Could you check a few things on this model? Use its own coordinates, in mm. Round coordinates to 2 decimals unless told otherwise and drop trailing zeros. Order: outer loops, then holes, each group sorted by start corner. A loop starts at its lowest first (then second) coordinate and runs counter-clockwise, first axis right, second up. Notation, with made-up numbers: (2, 42) - (56, 42) arc R8 cw to (56, 57) - close; hole circle Ø8 at (76.25, -30.75). An arc over 180 degrees is marked (long way). Return JSON: item names as keys, results as strings. Group by question number.
from build123d import *

# Parameters (mm, degrees)
EXTRUDE_1_DEPTH               = 104
SKETCH_2_W                    = 6
SKETCH_2_H                    = 104
CUT_EXTRUDE_1_DEPTH           = 21
HOLE_WIZARD_4_4_40_AT_2_COUNT = 2
HOLE_WIZARD_4_4_40_AT_2_PITCH = 10.2
HOLE_WIZARD_4_4_40_AT_3_COUNT = 2
HOLE_WIZARD_4_4_40_AT_3_PITCH = 48.876170063
HOLE_WIZARD_4_4_40_AT_4_COUNT = 2
HOLE_WIZARD_4_4_40_AT_4_PITCH = 47.8
HOLE_WIZARD_4_4_40_AT_5_COUNT = 2
HOLE_WIZARD_4_4_40_AT_5_PITCH = 24.438085031
SKETCH_6_W                    = 10
SKETCH_6_H                    = 28
CUT_EXTRUDE_3_DEPTH           = 3
HOLE_WIZARD_M31_AT_2_COUNT    = 2
HOLE_WIZARD_M31_AT_2_PITCH    = 42
HOLE_WIZARD_M31_AT_3_COUNT    = 2
HOLE_WIZARD_M31_AT_3_PITCH    = 90
HOLE_WIZARD_2_4_40_AT_2_COUNT = 2
HOLE_WIZARD_2_4_40_AT_2_PITCH = 34
SKETCH_13_W                   = 1.5
SKETCH_13_H                   = 37.2
CUT_EXTRUDE_6_DEPTH           = 54
HOLE_WIZARD_3_AT_2_COUNT      = 2
HOLE_WIZARD_3_AT_2_PITCH      = 12
HOLE_WIZARD_3_AT_3_COUNT      = 2
HOLE_WIZARD_3_AT_3_PITCH      = 7.071067812
HOLE_WIZARD_3_AT_4_COUNT      = 2
HOLE_WIZARD_3_AT_4_PITCH      = 29.83286778
CUT_EXTRUDE_8_DEPTH           = 2
SKETCH_18_R                   = 4
SKETCH_18_R_2                 = 1.4
CUT_EXTRUDE_9_DEPTH           = 3
CUT_EXTRUDE_10_REACH          = 4
SKETCH_19_R                   = 2.5


with BuildPart() as part:
    # Эскиз1 → Бобышка-Вытянуть1 (new body)
    with BuildSketch(Plane.XY):
        Polygon((0, 40), (0, 0), (20, 0), (20, 2), (2, 2), (2, 38), (10, 38), (10, 40), align=None)
    extrude(amount=EXTRUDE_1_DEPTH)

    # Эскиз2 → Вырез-Вытянуть1 (cut)
    with BuildSketch(Plane.XZ):
        with BuildLine():
            Line((5, 53), (0, 53))
            Line((0, 53), (0, 12))
            Line((0, 12), (5, 12))
            ThreePointArc((5, 12), (7.121320344, 12.878679656), (8, 15))
            Line((8, 15), (8, 50))
            ThreePointArc((8, 50), (7.121320344, 52.121320344), (5, 53))
        make_face()
        with Locations((17, 52)):
            Rectangle(SKETCH_2_W, SKETCH_2_H)
    extrude(amount=-CUT_EXTRUDE_1_DEPTH, mode=Mode.SUBTRACT)

    # Эскиз3 → 4_отв_4-40 (revolve, cut)
    with BuildSketch(Plane(origin=(0, 15.6, 8.6), x_dir=(0, 0, 1), z_dir=(0, 1, 0))):
        Polygon((0, 0), (0, 2), (1.651, 2), (1.0922, 1.4412), (1.0922, 0.5588), (1.651, 0), align=None)
    hole_wizard_4_4_40 = revolve(axis=Axis((-6.35, 15.6, 8.6), (1, 0, 0)), mode=Mode.SUBTRACT)

    # 4_отв_4-40 at 2: 4_отв_4-40 ×2
    with Locations(*[(0, -i * HOLE_WIZARD_4_4_40_AT_2_PITCH, 0) for i in range(1, HOLE_WIZARD_4_4_40_AT_2_COUNT)]):
        add(hole_wizard_4_4_40, mode=Mode.SUBTRACT)

    # 4_отв_4-40 at 3: 4_отв_4-40 ×2
    with Locations(*[Vector(0, -0.208690656, 0.977981702) * (i * HOLE_WIZARD_4_4_40_AT_3_PITCH) for i in range(1, HOLE_WIZARD_4_4_40_AT_3_COUNT)]):
        add(hole_wizard_4_4_40, mode=Mode.SUBTRACT)

    # 4_отв_4-40 at 4: 4_отв_4-40 ×2
    with Locations(*[(0, 0, i * HOLE_WIZARD_4_4_40_AT_4_PITCH) for i in range(1, HOLE_WIZARD_4_4_40_AT_4_COUNT)]):
        add(hole_wizard_4_4_40, mode=Mode.SUBTRACT)

    # 4_отв_4-40 at 5: 4_отв_4-40 ×2
    with Locations(*[Vector(0, -0.208690656, 0.977981702) * (i * HOLE_WIZARD_4_4_40_AT_5_PITCH) for i in range(1, HOLE_WIZARD_4_4_40_AT_5_COUNT)]):
        add(hole_wizard_4_4_40, mode=Mode.SUBTRACT)

    # Эскиз6 → Вырез-Вытянуть3 (cut)
    with BuildSketch(Plane(origin=(0, 40, 0), x_dir=(1, 0, 0), z_dir=(0, 1, 0))):
        with Locations((5, -21)):
            Rectangle(SKETCH_6_W, SKETCH_6_H)
    extrude(amount=-CUT_EXTRUDE_3_DEPTH, mode=Mode.SUBTRACT)

    # Эскиз8 → Отверстие с зазором M31 (revolve, cut)
    with BuildSketch(Plane(origin=(8.5, 0, 98), x_dir=(0, 0, -1), z_dir=(1, 0, 0))):
        Polygon((0, 0), (0, 2), (1.725, 2), (1.6, 1.875), (1.6, 0.125), (1.725, 0), align=None)
    hole_wizard_m31 = revolve(axis=Axis((8.5, -6.35, 98), (0, 1, 0)), mode=Mode.SUBTRACT)

    # Отверстие с зазором M31 at 2: Отверстие с зазором M31 ×2
    with Locations(*[(0, 0, -i * HOLE_WIZARD_M31_AT_2_PITCH) for i in range(1, HOLE_WIZARD_M31_AT_2_COUNT)]):
        add(hole_wizard_m31, mode=Mode.SUBTRACT)

    # Отверстие с зазором M31 at 3: Отверстие с зазором M31 ×2
    with Locations(*[(0, 0, -i * HOLE_WIZARD_M31_AT_3_PITCH) for i in range(1, HOLE_WIZARD_M31_AT_3_COUNT)]):
        add(hole_wizard_m31, mode=Mode.SUBTRACT)

    # Эскиз11 → 2_отв_4-40 (revolve, cut)
    with BuildSketch(Plane(origin=(5, 40, 38), x_dir=(0, 0, 1), z_dir=(1, 0, 0))):
        Polygon((0, 0), (0, 2), (1.651, 2), (1.0922, 1.4412), (1.0922, 0.5588), (1.651, 0), align=None)
    hole_wizard_2_4_40 = revolve(axis=Axis((5, 46.35, 38), (0, -1, 0)), mode=Mode.SUBTRACT)

    # 2_отв_4-40 at 2: 2_отв_4-40 ×2
    with Locations(*[(0, 0, -i * HOLE_WIZARD_2_4_40_AT_2_PITCH) for i in range(1, HOLE_WIZARD_2_4_40_AT_2_COUNT)]):
        add(hole_wizard_2_4_40, mode=Mode.SUBTRACT)

    # Эскиз13 → Вырез-Вытянуть6 (cut)
    with BuildSketch(Plane.XY.offset(104)):
        with Locations((4.75, 20)):
            Rectangle(SKETCH_13_W, SKETCH_13_H)
    extrude(amount=-CUT_EXTRUDE_6_DEPTH, mode=Mode.SUBTRACT)

    # Эскиз15 → М3 потай (revolve, cut)
    with BuildSketch(Plane(origin=(2, 34, 89), x_dir=(0, 0, -1), z_dir=(0, 1, 0))):
        Polygon((0, 0), (0, 2), (1.8, 2), (1.7, 1.9), (1.7, 1.3), (3, 0), align=None)
    hole_wizard_3 = revolve(axis=Axis((8.35, 34, 89), (-1, 0, 0)), mode=Mode.SUBTRACT)

    # М3 потай at 2: М3 потай ×2
    with Locations(*[(0, -i * HOLE_WIZARD_3_AT_2_PITCH, 0) for i in range(1, HOLE_WIZARD_3_AT_2_COUNT)]):
        add(hole_wizard_3, mode=Mode.SUBTRACT)

    # М3 потай at 3: М3 потай ×2
    with Locations(*[Vector(0, 0.141421356, 0.989949494) * (i * HOLE_WIZARD_3_AT_3_PITCH) for i in range(1, HOLE_WIZARD_3_AT_3_COUNT)]):
        add(hole_wizard_3, mode=Mode.SUBTRACT)

    # М3 потай at 4: М3 потай ×2
    with Locations(*[Vector(0, -0.972082209, 0.234640533) * (i * HOLE_WIZARD_3_AT_4_PITCH) for i in range(1, HOLE_WIZARD_3_AT_4_COUNT)]):
        add(hole_wizard_3, mode=Mode.SUBTRACT)

    # Эскиз17 → Вырез-Вытянуть8 (cut)
    with BuildSketch(Plane.XZ):
        Polygon((0, 104), (2.828427125, 104), (0, 101.171572875), align=None)
    extrude(amount=-CUT_EXTRUDE_8_DEPTH, mode=Mode.SUBTRACT)

    # Эскиз18 → Вырез-Вытянуть9 (cut, through all)
    with BuildSketch(Plane(origin=(2, 0, 0), x_dir=(0, 0, -1), z_dir=(1, 0, 0))):
        with BuildLine():
            Line((-7, 30), (-7, 37))
            Line((-7, 37), (-15, 37))
            Line((-15, 37), (-15, 30))
            ThreePointArc((-15, 30), (-11, 26), (-7, 30))
        make_face()
        with Locations((-42, 26)):
            Circle(SKETCH_18_R)
        with Locations((-50, 26)):
            Circle(SKETCH_18_R_2)
        with Locations((-34, 26)):
            Circle(SKETCH_18_R_2)
    extrude(amount=-CUT_EXTRUDE_9_DEPTH, mode=Mode.SUBTRACT)

    # Эскиз19 → Вырез-Вытянуть10 (cut, up to next)
    with BuildSketch(Plane(origin=(2, 0, 0), x_dir=(0, 0, -1), z_dir=(1, 0, 0)), mode=Mode.PRIVATE) as cut_extrude_10_sk1:
        with Locations((-95, 13.5)):
            Circle(SKETCH_19_R)
    cut_extrude_10_tool1 = extrude(cut_extrude_10_sk1.sketch, amount=-CUT_EXTRUDE_10_REACH, mode=Mode.PRIVATE) & part.part
    add(cut_extrude_10_tool1.solids().sort_by_distance((2, 13.5, 95))[0], mode=Mode.SUBTRACT)


solid = part.part
1) I want a section at C-C, the plane z = 77.5. List the corners of the cut face in (x, y) for me, plus the area to 3 significant figures.
2) Will these pins go through, and if not, where does the flat tip stop? pin 1 (2 mm diameter, centred on y = 5, z = 96, fed in from +X); pin 2 (2.5 mm diameter, centred on x = 8.5, z = 8, fed in from -Y); pin 3 (12 mm diameter, centred on y = 20, z = 45.5, fed in from +X).
3) I want a section at A-A, the plane z = 42. List the corners of the cut face in (x, y) for me.
4) I want a section at B-B, the plane y = 28.5. List the corners of the cut face in (x, z) for me.
5) If I drill on line 1 along Y through (x, z) = (1.25, 56.4); line 2 along Z through (x, y) = (8.5, 1.1); line 3 along Y through (x, z) = (0.3, 89), over which ranges is the centre line in solid material (lowest first)? Write a range as from..to.
Outcome:
{
 "1": {"outline": "(0, 0) - (14, 0) - (14, 2) - (5.5, 2) - (5.5, 1.4) - (4, 1.4) - (4, 2) - (2, 2) - (2, 38) - (4, 38) - (4, 38.6) - (5.5, 38.6) - (5.5, 38) - (10, 38) - (10, 40) - (0, 40) - close", "area": "118 mm^2"},
 "2": {"pin 1": "through", "pin 2": "y = 38", "pin 3": "x = 2"},
 "3": {"outline": "(0, 21) - (2, 21) - (2, 22) - (0, 22) - close; (0, 30) - (2, 30) - (2, 38) - (10, 38) - (10, 40) - (0, 40) - close; (8, 0) - (14, 0) - (14, 2) - (8, 2) - close"},
 "4": {"outline": "(0, 0) - (2, 0) - (2, 7.29) - (0, 7.29) - close; (0, 14.71) - (2, 14.71) - (2, 38.88) - (0, 38.88) - close; (0, 45.12) - (2, 45.12) - (2, 104) - (0, 104) - close"},
 "5": {"line 1": "0..4.31, 6.49..14.51, 16.69..40", "line 2": "0..6.4, 9.6..54.4, 57.6..96.4, 99.6..104", "line 3": "0..20.3, 23.7..32.3, 35.7..40"}
}
